Design review of the part built by this model. Coordinates are the model's own, in mm. A direction names the side the tool comes from. Round coordinates to 2 decimals unless told otherwise and drop trailing zeros. Write each loop counter-clockwise with the first axis right and the second up, starting at its lowest first coordinate (ties: lowest second). Pieces come first, ordered by that corner, then holes. Notation, with made-up numbers: M 63,65 L 82,65 A10 cw 82,80 Z; hole C 36.25,-11.75 d10. An arc over 180 degrees is marked long. Use CSV: the item, a comma, the result in double quotes.
from build123d import *

# Parameters (mm, degrees)
F2_W     = 60
F2_H     = 91
F3_DEPTH = 10
F4_W     = 56
F4_H     = 87
F5_DEPTH = 8
F6_R     = 4
F7_DEPTH = 10
F8_R     = 2
F9_DEPTH = 10.001


with BuildPart() as f3:
    # F2 (on Top) → F3 (new body)
    with BuildSketch(Plane.XY):
        Rectangle(F2_W, F2_H)
    extrude(amount=F3_DEPTH)

    # F4 (on face) → F5 (cut)
    with BuildSketch(Plane.XY.offset(10)):
        Rectangle(F4_W, F4_H)
    extrude(amount=-F5_DEPTH, mode=Mode.SUBTRACT)

    # F6 (on face) → F7 (join)
    with BuildSketch(Plane(origin=(0, 0, 0), x_dir=(1, 0, 0), z_dir=(0, 0, -1))):
        with Locations((0, -41.5)):
            Circle(F6_R)
        with Locations((0, 41.5)):
            Circle(F6_R)
    extrude(amount=-F7_DEPTH)

    # F8 (on face) → F9 (cut, through all)
    with BuildSketch(Plane(origin=(0, 0, 0), x_dir=(1, 0, 0), z_dir=(0, 0, -1))):
        with Locations((0, -41.5)):
            Circle(F8_R)
        with Locations((0, 41.5)):
            Circle(F8_R)
    extrude(amount=-F9_DEPTH, mode=Mode.SUBTRACT)


solid = f3.part
1) The part is to be moulded in two halves that separate along Y. For faces 3 (the face through (-30, -1, 5)), 4 (the face through (-0.1, -37.5, 5.9)), 5 (the face through (0, -45.5, 5)), say which applies: released by +Y, released by -Y, zero draft, split by the parting line, or undercut.
Answers:
face 3,"zero draft"
face 4,"undercut"
face 5,"released by -Y"
2) Add section B-B on z = 3.25. Write out the cut boundary in (x, y).
Answers:
outline,"M -30,-45.5 L 30,-45.5 L 30,45.5 L -30,45.5 Z; hole M -28,-43.5 L -3.46,-43.5 A4 cw long 3.46,-43.5 L 28,-43.5 L 28,43.5 L 3.46,43.5 A4 cw long -3.46,43.5 L -28,43.5 Z; hole C 0,-41.5 d4; hole C 0,41.5 d4"
3) Wall thickness on line 1 along Y through (x, z) = (0, 3); line 2 along X through (y, z) = (41.5, 6); line 3 along Y through (x, z) = (-17.5, 5.25): over which ranges is each line inside the solid? List them lowest first. Write a range as [from, to].
Answers:
line 1,"[-45.5, -43.5], [-39.5, -37.5], [37.5, 39.5], [43.5, 45.5]"
line 2,"[-30, -28], [-4, -2], [2, 4], [28, 30]"
line 3,"[-45.5, -43.5], [43.5, 45.5]"
4) Add section D-D on x = -20.5. Write out the cut boundary in (y, z).
Answers:
outline,"M -45.5,0 L 45.5,0 L 45.5,10 L 43.5,10 L 43.5,2 L -43.5,2 L -43.5,10 L -45.5,10 Z"
5) Add section C-C on x = 0. Write out the cut boundary in (y, z), then the cut area to 3 significant figures.
Answers:
outline,"M -45.5,0 L -43.5,0 L -43.5,10 L -45.5,10 Z; M -39.5,0 L 39.5,0 L 39.5,10 L 37.5,10 L 37.5,2 L -37.5,2 L -37.5,10 L -39.5,10 Z; M 43.5,0 L 45.5,0 L 45.5,10 L 43.5,10 Z"
area,"230 mm²"
6) Machinability: for faces 1 (the face through (-29, 4, 10)), 2 (the face through (0, 1, 2)), which of the approach directions +Z, -Z, +X, -X, +Y, -Y give a long, thin tool a straight path to every point of the face, cutting with its end or side? Answer none if there is none.
Answers:
face 1,"+Z, +X, -X, +Y, -Y"
face 2,"+Z"
7) For pin 1 Ø6.5 at (x, y) = (0, -41.5) entering from -Z; pin 2 Ø3.5 at (x, y) = (0, 41.5) entering from +Z, all flat-tipped, find the tip position at first contact; note any pin that passes through.
Answers:
pin 1,"z = 0"
pin 2,"through"
8) Add section A-A on y = 41.5. Write out the cut boundary in (x, z), then the cut area to 3 significant figures.
Answers:
outline,"M -30,0 L -2,0 L -2,10 L -4,10 L -4,2 L -28,2 L -28,10 L -30,10 Z; M 2,0 L 30,0 L 30,10 L 28,10 L 28,2 L 4,2 L 4,10 L 2,10 Z"
area,"176 mm²"
